```python
from build123d import *

# Parameters (mm, degrees)
F0_W        = 55
F0_H        = 450
F1_DEPTH    = 22
F2_W        = 55
F2_H        = 1.5
F3_DEPTH    = 7
F4_W        = 3
F4_H        = 375
F5_DEPTH    = 55.001
F6_T1_DEPTH = 55
F7_R        = 40


# Not quite as in the source:
# - a fillet or chamfer that OpenCascade refuses, or shapes differently, is made with other operations: its cross-section is extruded or revolved along the edge and cut away or added


with BuildPart() as f1:
    # F0 (on Front) → F1 (new body)
    with BuildSketch(Plane.XZ):
        Rectangle(F0_W, F0_H)
    extrude(amount=F1_DEPTH)

    # F2 (on face) → F3 (join)
    with BuildSketch(Plane(origin=(0, 0, -225), x_dir=(1, 0, 0), z_dir=(0, 0, -1))):
        with Locations((0, 21.25)):
            Rectangle(F2_W, F2_H)
    extrude(amount=F3_DEPTH)

    # F4 (on face) → F5 (cut, through all)
    with BuildSketch(Plane(origin=(-27.5, 0, 0), x_dir=(0, -1, 0), z_dir=(-1, 0, 0))):
        with Locations((1.5, 37.5)):
            Rectangle(F4_W, F4_H)
    extrude(amount=-F5_DEPTH, mode=Mode.SUBTRACT)

    # F6: fillet of radius 5 on 1 edges, made by hand

    # F6_s2 → F6_t1 (join)
    with BuildSketch(Plane.YZ.offset(-27.5)):
        with BuildLine():
            ThreePointArc((-3, -145.417424305), (-2.1833001327, -148.1560370926), (0, -150))
            Line((0, -150), (-3, -150))
            Line((-3, -150), (-3, -145.417424305))
        make_face()
    extrude(amount=F6_T1_DEPTH)

    # F7
    f7_edges = [f1.edges().sort_by_distance(p)[0] for p in [
        (0, 0, -150),
    ]]
    fillet(f7_edges, radius=F7_R)


solid = f1.part
```
Design review of the part built by this model. Coordinates are the model's own, in mm. A direction names the side the tool comes from. Coordinates: 2 decimals unless noted, no trailing zeros. Write each loop counter-clockwise with the first axis right and the second up, starting at its lowest first coordinate (ties: lowest second). Pieces come first, ordered by that corner, then holes.
1) To check wall thickness, follow L1, parallel to Y at x = 13.5, z = 41; L2, parallel to Z at x = -18, y = -9.25. State the ranges of each line that lie inside material, in increasing order.
2) Add section A-A (x = -18.5). Write out the cut boundary in (y, z), plus the area to 3 significant figures.
3) Machinability: for faces 1 (the flat face through (0, -10, -225)), 2 (the flat face through (0, -3, 37)), 3 (the flat face through (0, -12, 225)), which of the approach directions +Z, -Z, +X, -X, +Y, -Y give a long, thin tool a straight path to every point of the face, cutting with its end or side? Answer none if there is none.
4) Add section B-B (y = -12.75). Write out the cut boundary in (x, z).
5) Insertion check: pin 1 (8 mm diameter, centred on x = 2, z = 133.5, fed in from +Y); pin 2 (2 mm diameter, centred on x = -1, y = -3.5, fed in from -Z); pin 3 (5.5 mm diameter, centred on x = -1.5, z = -228, fed in from +Y). Each pin has a flat end and moves straight along its axis. Give the tip position at first contact, or say it passes through.
6) Add section C-C (z = 39.5). Write out the cut boundary in (x, y), plus the area to 4 significant figures.
Check result:
1. L1: y = -22 to -3
1. L2: z = -225 to 225
2. outline: (-22, -232) - (-20.5, -232) - (-20.5, -225) - (0, -225) - (0, -161.57) arc R40 ccw to (-2.67, -147.21) arc R5 cw to (-3, -145.42) - (-3, 225) - (-22, 225) - close
2. area: 8,780 mm2
3. face 1: -Z, +X, -X, +Y
3. face 2: +Z, +X, -X, +Y
3. face 3: +Z, +X, -X, +Y, -Y
4. outline: (-27.5, -225) - (27.5, -225) - (27.5, 225) - (-27.5, 225) - close
5. pin 1: stops at y = -3
5. pin 2: stops at z = -225
5. pin 3: stops at y = -20.5
6. outline: (-27.5, -22) - (27.5, -22) - (27.5, -3) - (-27.5, -3) - close
6. area: 1,045 mm2
